The model under review builds one solid part; all positions refer to its coordinate system, in mm. A direction names the side the tool comes from. Coordinates: 2 decimals unless noted, no trailing zeros. Loops run counter-clockwise (first coordinate to the right, second up) from the corner with the lowest first, then second, coordinate; pieces in that order, holes last. Notation, with made-up numbers: M -30,58.5 L -14,58.5 A17 cw -14,69.5 Z; hole C 59.5,-28.5 d6. An arc over 180 degrees is marked long. Return JSON: item names as keys, results as strings.
```python
from build123d import *

# Parameters (mm, degrees)
F0_R     = 15
F0_R_2   = 11
F1_DEPTH = 10
F0_R_3   = 44
F2_DEPTH = 2
F3_R     = 2
F4_DEPTH = 25


with BuildPart() as f1:
    # F0 (on Top) → F1 (new body)
    with BuildSketch(Plane.XY):
        Circle(F0_R)
        Circle(F0_R_2, mode=Mode.SUBTRACT)
    extrude(amount=F1_DEPTH)

    # F0 (on Top) → F2 (join)
    with BuildSketch(Plane.XY):
        Circle(F0_R_3)
        Circle(F0_R, mode=Mode.SUBTRACT)
    extrude(amount=F2_DEPTH)

    # F3 (on Right) → F4 (cut, symmetric)
    with BuildSketch(Plane.YZ):
        with Locations((0, 5.560728)):
            Circle(F3_R)
    extrude(amount=F4_DEPTH, both=True, mode=Mode.SUBTRACT)


solid = f1.part
```
1. Add section A-A on x = 0. Give the boundary of the cut face in (y, z).
Check values:
{"outline": "M -44,0 L -11,0 L -11,10 L -15,10 L -15,2 L -44,2 Z; M 11,0 L 44,0 L 44,2 L 15,2 L 15,10 L 11,10 Z"}
2. Add section D-D on x = -12. Give the boundary of the cut face in (y, z).
Check values:
{"outline": "M -42.33,0 L 42.33,0 L 42.33,2 L 9,2 L 9,10 L -9,10 L -9,2 L -42.33,2 Z; hole C 0,5.56 d4"}
3. To check wall thickness, follow line 1 (Y direction, x = 0, z = 3.25); line 2 (Z direction, x = 11, y = -11); line 3 (X direction, y = 10, z = 4.5). State the ranges of each line that lie inside material, in increasing order.
Check values:
{"line 1": "-15 to -11, 11 to 15", "line 2": "0 to 2", "line 3": "-11.18 to -4.58, 4.58 to 11.18"}
4. Insertion check: pin 1 Ø3 at (y, z) = (27, 3) entering from -X; pin 2 Ø1 at (x, z) = (23.5, 1) entering from +Y; pin 3 Ø4 at (x, y) = (-35, 4) entering from +Z. Each pin has a flat end and moves straight along its axis. Give the tip position at first contact, or say it passes through.
Check values:
{"pin 1": "x = -35.58", "pin 2": "y = 37.51", "pin 3": "z = 2"}
5. Add section B-B on y = 0. Give the boundary of the cut face in (x, z).
Check values:
{"outline": "M -44,0 L -11,0 L -11,3.56 L -15,3.56 L -15,2 L -44,2 Z; M -15,7.56 L -11,7.56 L -11,10 L -15,10 Z; M 11,0 L 44,0 L 44,2 L 15,2 L 15,3.56 L 11,3.56 Z; M 11,7.56 L 15,7.56 L 15,10 L 11,10 Z"}
6. Add section C-C on z = 8.75. Give the boundary of the cut face in (x, y), plus the area to 3 significant figures.
Check values:
{"outline": "C 0,0 d30; hole C 0,0 d22", "area": "327 mm²"}
7. The part is to be moulded in two halves that separate along Y. For faces 3 (the face through (9, -9, 0)), 4 (the face through (14.307, 4.506, 5.944)), 5 (the face through (10.161, -4.213, 4.93)), say which applies: released by +Y, released by -Y, zero draft, split by the parting line, or undercut.
Check values:
{"face 3": "zero draft", "face 4": "split by the parting line", "face 5": "undercut"}
8. Machinability: for faces 1 (the face through (-9.538, -42.954, 0.986)), 2 (the face through (-1, -19, 2)), which of the approach directions +Z, -Z, +X, -X, +Y, -Y give a long, thin tool a straight path to every point of the face, cutting with its end or side? Answer none if there is none.
Check values:
{"face 1": "+Z, -Z", "face 2": "+Z"}
